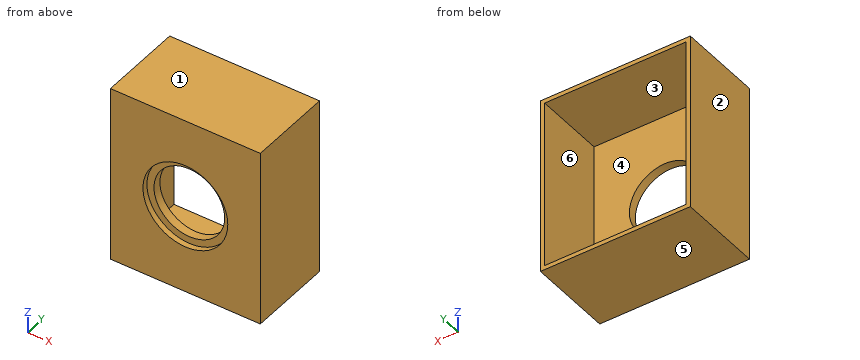
Autodesk Inventor part; units mm, degrees
ref_plane "YZ Plane" through (0, 0, 0) normal (1, 0, 0) x (0, 1, 0)
ref_plane "XZ Plane" through (0, 0, 0) normal (0, 1, 0) x (-1, 0, 0)
ref_plane "XY Plane" through (0, 0, 0) normal (0, 0, 1) x (1, 0, 0)
sketch "Sketch1" plane through (0, 0, 0) normal (0, 1, 0) x (-1, 0, 0)
  line L0 (26.5, 31.5) -> (-26.5, 31.5)
  line L1 (-26.5, 31.5) -> (-26.5, -31.5)
  line L2 (-26.5, -31.5) -> (26.5, -31.5)
  line L3 (26.5, -31.5) -> (26.5, 31.5)
  line L4 (26.5, 31.5) -> (-26.5, -31.5) construction
  line L5 (-26.5, 31.5) -> (26.5, -31.5) construction
  point P0 (0, 0)
  dimension "d0" = 53
  dimension "d1" = 63
extrude "Extrusion1" add sketch "Sketch1" along normal blind 30
sketch "Sketch2" plane through (0, 30, 0) normal (0, 1, 0) x (1, 0, 0)
  line L0 (-25, -30) -> (25, -30)
  line L1 (25, -30) -> (25, 30)
  line L2 (25, 30) -> (-25, 30)
  line L3 (-25, 30) -> (-25, -30)
  line L4 (-25, -30) -> (25, 30) construction
  line L5 (25, -30) -> (-25, 30) construction
  point P0 (0, 0)
  dimension "d4" = 50
  dimension "d5" = 60
extrude "Extrusion2" cut sketch "Sketch2" against normal blind 25
sketch "Sketch3" plane through (0, 0, 0) normal (0, -1, 0) x (1, 0, 0)
  line L0 (26.5, -31.5) -> (-26.5, -31.5)
  circle A0 centre (0, 0) radius 15
  dimension "d10" = 30
extrude "Extrusion3" cut sketch "Sketch3" against normal blind 2
sketch "Sketch4" plane through (0, 2, 0) normal (0, -1, 0) x (1, 0, 0)
  circle A0 centre (0, 0) radius 12.5
  dimension "d13" = 25
extrude "Extrusion4" cut sketch "Sketch4" against normal up to next
properties part number "cover"
Geometry: final body of the model. Coordinates: model frame, mm. Face numbers are marked on the shaded views. A direction names the side the tool comes from. Coordinates: 2 decimals unless noted, no trailing zeros. Loops run counter-clockwise (first coordinate to the right, second up) from the corner with the lowest first, then second, coordinate; pieces in that order, holes last. Notation, with made-up numbers: M 32,30 L 91,30 A23 ccw 91,45 Z; hole C 70,-7 d2. An arc over 180 degrees is marked long. Put each result on its own line as item: value.
(1) First-contact query: pin 1 (24 mm diameter, centred on x = 0, z = 0, fed in from -Y); pin 2 (8 mm diameter, centred on x = -10, z = 7, fed in from +Y). Flat tips, straight axial feed; report the tip coordinate or a pass-through.
Answer sheet:
pin 1: passes through
pin 2: stops at y = 5
(2) Cut plane C-C on y = 22.25. Return the cut outline in (x, z).
Answer sheet:
outline: M -26.5,-31.5 L 26.5,-31.5 L 26.5,31.5 L -26.5,31.5 Z; hole M -25,-30 L 25,-30 L 25,30 L -25,30 Z
(3) Cut plane A-A on z = 0. Return the cut outline in (x, y).
Answer sheet:
outline: M -26.5,0 L -15,0 L -15,2 L -12.5,2 L -12.5,5 L -25,5 L -25,30 L -26.5,30 Z; M 12.5,2 L 15,2 L 15,0 L 26.5,0 L 26.5,30 L 25,30 L 25,5 L 12.5,5 Z
(4) Cut plane D-D on z = -18.5. Return the cut outline in (x, y), then the cut area to 3 significant figures.
Answer sheet:
outline: M -26.5,0 L 26.5,0 L 26.5,30 L 25,30 L 25,5 L -25,5 L -25,30 L -26.5,30 Z
area: 340 mm^2
(5) Material intervals for probe 1 along Z at (x, y) = (-13, 6.25); probe 2 along X at (y, z) = (15.5, 18); probe 3 along Z at (x, y) = (0, 1.6), sorted ascending.
Answer sheet:
probe 1: z = -31.5 to -30, 30 to 31.5
probe 2: x = -26.5 to -25, 25 to 26.5
probe 3: z = -31.5 to -15, 15 to 31.5
(6) Access query for the marked faces 5 and 6. Directions: +Z, -Z, +X, -X, +Y, -Y. A direction counts if a zero-diameter tool reaches every point of the face in a straight line with its end or side. Return the directions, or none.
Answer sheet:
face 5: -Z, +X, -X, +Y, -Y
face 6: +Y
(7) Cut plane B-B on x = 0. Return the cut outline in (y, z), then the cut area to 3 significant figures.
Answer sheet:
outline: M 0,-31.5 L 30,-31.5 L 30,-30 L 5,-30 L 5,-12.5 L 2,-12.5 L 2,-15 L 0,-15 Z; M 0,15 L 2,15 L 2,12.5 L 5,12.5 L 5,30 L 30,30 L 30,31.5 L 0,31.5 Z
area: 255 mm^2
(8) Draft query along X for the marked faces 1, 2, 3 and 4. Return one class per face: pulls with the +X half, pulls with the -X half, needs draft (parallel to the pull), parting line crosses it, or undercut.
Answer sheet:
face 1: needs draft
face 2: pulls with the -X half
face 3: undercut
face 4: undercut
